For this review, take the finished solid that the model builds, in its own axes (mm). Round coordinates to 2 decimals unless told otherwise and drop trailing zeros. Order: outer loops, then holes, each group sorted by start corner. A loop starts at its lowest first (then second) coordinate and runs counter-clockwise, first axis right, second up. Notation, with made-up numbers: (-13.5, 54) - (8.5, 54) arc R8 ccw to (8.5, 62) - close; hole circle Ø10 at (-24.75, 39). An arc over 180 degrees is marked (long way). One line per question, with ' | ' between items.
```python
from build123d import *

# Parameters (mm, degrees)
SKETCH_1_W          = 6
SKETCH_1_H          = 6
EXTRUDE_1_DEPTH     = 78
SKETCH_2_R          = 1.2
SKETCH_2_R_2        = 1
CUT_EXTRUDE_1_DEPTH = 80
SKETCH_3_R          = 1.2
CUT_EXTRUDE_2_DEPTH = 80


with BuildPart() as part:
    # 草图1 → 凸台-拉伸1 (new body)
    with BuildSketch(Plane.XY):
        with Locations((3, 3)):
            Rectangle(SKETCH_1_W, SKETCH_1_H)
    extrude(amount=EXTRUDE_1_DEPTH)

    # 草图2 → 切除-拉伸1 (cut)
    with BuildSketch(Plane(origin=(0, 6, 0), x_dir=(1, 0, 0), z_dir=(0, 1, 0))):
        with Locations(Location((3, -74, 0), (0, 0, 270))):
            Circle(SKETCH_2_R)
        with Locations(Location((3, -4, 0), (0, 0, 270))):
            Circle(SKETCH_2_R)
        with Locations(Location((3, -12, 0), (0, 0, 270))):
            Circle(SKETCH_2_R_2)
        with Locations(Location((3, -66, 0), (0, 0, 270))):
            Circle(SKETCH_2_R_2)
    extrude(amount=-CUT_EXTRUDE_1_DEPTH, mode=Mode.SUBTRACT)

    # 草图3 → 切除-拉伸2 (cut)
    with BuildSketch(Plane(origin=(6, 0, 0), x_dir=(0, 0, -1), z_dir=(1, 0, 0))):
        with Locations((-60, 3)):
            Circle(SKETCH_3_R)
        with Locations((-18, 3)):
            Circle(SKETCH_3_R)
    extrude(amount=-CUT_EXTRUDE_2_DEPTH, mode=Mode.SUBTRACT)


solid = part.part
```
(1) Mouldability with a two-part tool opening along X and no side actions: class faces 1 (the cylindrical face through (4.01, 3.04, 4.65)), 2 (the flat face through (0, 3, 38)), 3 (the cylindrical face through (3.04, 3.05, 19.2)), 4 (the cylindrical face through (3, 3, 65)) as released by +X, released by -X, zero draft, split by the parting line, or undercut.
Output values:
face 1: undercut | face 2: released by -X | face 3: zero draft | face 4: undercut
(2) We need section D-D on z = 4. State the section outline as (x, y) points.
Output values:
outline: (0, 0) - (1.8, 0) - (1.8, 6) - (0, 6) - close; (4.2, 0) - (6, 0) - (6, 6) - (4.2, 6) - close
(3) For probe 1 along X at (y, z) = (4.35, 12); probe 2 along Z at (x, y) = (0.7, 2.3); probe 3 along Y at (x, z) = (2, 18), list the stretches that pass through material, from the lowest coordinate up. Write a range as [from, to].
Output values:
probe 1: [0, 2], [4, 6] | probe 2: [0, 17.03], [18.97, 59.03], [60.97, 78] | probe 3: [0, 1.8], [4.2, 6]
(4) We need section C-C on x = 1. State the section outline as (y, z) points.
Output values:
outline: (0, 0) - (6, 0) - (6, 78) - (0, 78) - close; hole circle Ø2.4 at (3, 18); hole circle Ø2.4 at (3, 60)
(5) Insertion check: pin 1 (2.5 mm diameter, centred on x = 3, z = 12, fed in from -Y); pin 2 (1.9 mm diameter, centred on y = 3, z = 18, fed in from +X). Each pin has a flat end and moves straight along its axis. Give the tip position at first contact, or say it passes through.
Output values:
pin 1: y = 0 | pin 2: through
(6) We need section A-A on z = 12. State the section outline as (x, y) points.
Output values:
outline: (0, 0) - (2, 0) - (2, 6) - (0, 6) - close; (4, 0) - (6, 0) - (6, 6) - (4, 6) - close
(7) We need section B-B on y = 3. State the section outline as (x, z) points.
Output values:
outline: (0, 0) - (6, 0) - (6, 16.8) - (0, 16.8) - close; (0, 19.2) - (6, 19.2) - (6, 58.8) - (0, 58.8) - close; (0, 61.2) - (6, 61.2) - (6, 78) - (0, 78) - close; hole circle Ø2.4 at (3, 4); hole circle Ø2.4 at (3, 74); hole circle Ø2 at (3, 12); hole circle Ø2 at (3, 66)
